Can you work these out from the model? Positions are in its coordinate system, mm. A direction names the side the tool comes from. Give positions to 0.01 mm unless a question says otherwise; leave off trailing zeros. Order: outer loops, then holes, each group sorted by start corner. A loop starts at its lowest first (then second) coordinate and runs counter-clockwise, first axis right, second up. Notation, with made-up numbers: (-22, 21) - (2, 21) arc R34 cw to (2, 55) - close; hole circle Ø5 at (-21, -33.5). An arc over 180 degrees is marked (long way). Answer as CSV lines item,"result".
```python
from build123d import *

# Parameters (mm, degrees)
SKETCH1_R           = 1.5875
BOSS_EXTRUDE1_DEPTH = 0.889
SKETCH2_R           = 1.9685
BOSS_EXTRUDE2_DEPTH = 6.35
SKETCH4_W           = 3.2512
SKETCH4_H           = 3.2512
BOSS_EXTRUDE3_DEPTH = 5.08
SKETCH5_R           = 0.9271
CUT_EXTRUDE1_DEPTH  = 5.08


with BuildPart() as part:
    # Sketch1 → Boss-Extrude1 (new body)
    with BuildSketch(Plane.XY):
        Circle(SKETCH1_R)
    extrude(amount=BOSS_EXTRUDE1_DEPTH)

    # Sketch2 → Boss-Extrude2 (add)
    with BuildSketch(Plane.XY.offset(0.889)):
        Circle(SKETCH2_R)
    extrude(amount=BOSS_EXTRUDE2_DEPTH)

    # Sketch4 → Boss-Extrude3 (add)
    with BuildSketch(Plane.XY.offset(7.239)):
        Rectangle(SKETCH4_W, SKETCH4_H)
    extrude(amount=BOSS_EXTRUDE3_DEPTH)

    # Sketch5 → Cut-Extrude1 (cut)
    with BuildSketch(Plane.XY.offset(12.319)):
        Circle(SKETCH5_R)
    extrude(amount=-CUT_EXTRUDE1_DEPTH, mode=Mode.SUBTRACT)


solid = part.part
```
1) I want a section at A-A on y = 0. Write out the boundary of the cut face in (x, z), plus the area to 3 significant figures.
Answer block:
outline,"(-1.97, 0.89) - (-1.59, 0.89) - (-1.59, 0) - (1.59, 0) - (1.59, 0.89) - (1.97, 0.89) - (1.97, 7.24) - (1.63, 7.24) - (1.63, 12.32) - (0.93, 12.32) - (0.93, 7.24) - (-0.93, 7.24) - (-0.93, 12.32) - (-1.63, 12.32) - (-1.63, 7.24) - (-1.97, 7.24) - close"
area,"34.9 mm2"
2) Which directions (+Z, -Z, +X, -X, +Y, -Y) give clear straight access to the entire face, cutting with the end or side of a thin tool? Please do faces 1 (the flat face through (1.626, 0, 10)), 2 (the cylindrical face through (-0.43, -1.92, 4.02)), 3 (the flat face through (0, 1.626, 10)).
Answer block:
face 1,"+Z, +X, +Y, -Y"
face 2,"-Z"
face 3,"+Z, +X, -X, +Y"
3) If we mould it in two halves opening along X, with no side actions, what happens to faces 4 (the flat face through (0, 0, 7.239)), 5 (the flat face through (-1.626, 0, 10)), 6 (the flat face through (0, -1.626, 10)), 7 (the cylindrical face through (0.43, -0.82, 9.81))? For each: +X half, -X half, draft (parallel to the pull), parting line (faces both ways), or undercut.
Answer block:
face 4,"undercut"
face 5,"-X half"
face 6,"draft"
face 7,"undercut"
4) I'm going to push flat-ended pins straight in: P1, Ø1, axis at x = 0, z = 10, coming from the +Y side; P2, Ø1.6, axis at y = 0, z = 9.5, coming from the +X side; P3, Ø0.9, axis at x = 0, y = 0, coming from the +Z side. Where does each tip first touch, or does it pass through?
Answer block:
P1,"y = 1.63"
P2,"x = 1.63"
P3,"z = 7.24"
5) I need wall thicknesses on line 1 along Y through (x, z) = (0, 10.9); line 2 along Z through (x, y) = (-0.6, 0.15); line 3 along Y through (x, z) = (-0.1, 2.5). Which ranges of each line are inside material? Lowest first, please. Write a range as [from, to].
Answer block:
line 1,"[-1.63, -0.93], [0.93, 1.63]"
line 2,"[0, 7.24]"
line 3,"[-1.97, 1.97]"
6) I want a section at D-D on z = 6.5. Write out the boundary of the cut face in (x, y).
Answer block:
outline,"circle Ø3.94 at (0, 0)"
7) I want a section at B-B on z = 11.75. Write out the boundary of the cut face in (x, y).
Answer block:
outline,"(-1.63, -1.63) - (1.63, -1.63) - (1.63, 1.63) - (-1.63, 1.63) - close; hole circle Ø1.85 at (0, 0)"
